Can you work these out from the model? Positions are in its coordinate system, mm. Round coordinates to 2 decimals unless told otherwise and drop trailing zeros. Loops run counter-clockwise (first coordinate to the right, second up) from the corner with the lowest first, then second, coordinate; pieces in that order, holes last. Notation, with made-up numbers: (46, -35.75) - (95, -35.75) arc R28 cw to (95, -12.75) - close; hole circle Ø11 at (-25.75, 59.25). An arc over 180 degrees is marked (long way). Answer as CSV lines item,"result".
```python
from build123d import *

# Parameters (mm, degrees)
F0_W     = 1219.2
F0_H     = 76.2
F1_DEPTH = 38.1
F3_DEPTH = 38.101
F4_R     = 5.08


with BuildPart() as f1:
    # F0 (on Top) → F1 (new body)
    with BuildSketch(Plane.XY):
        Rectangle(F0_W, F0_H)
    extrude(amount=F1_DEPTH)

    # F2 (on face) → F3 (cut, through all)
    with BuildSketch(Plane.XY.offset(38.1)):
        Polygon((-609.6, 38.1), (-609.6, -38.1), (-533.4, 38.1), align=None)
        Polygon((533.4, 38.1), (609.6, -38.1), (609.6, 38.1), align=None)
    extrude(amount=-F3_DEPTH, mode=Mode.SUBTRACT)

    # F4
    f4_edges = [f1.edges().sort_by_distance(p)[0] for p in [
        (0, 38.1, 0),
        (0, -38.1, 0),
        (0, -38.1, 38.1),
        (0, 38.1, 38.1),
    ]]
    fillet(f4_edges, radius=F4_R)


solid = f1.part
```
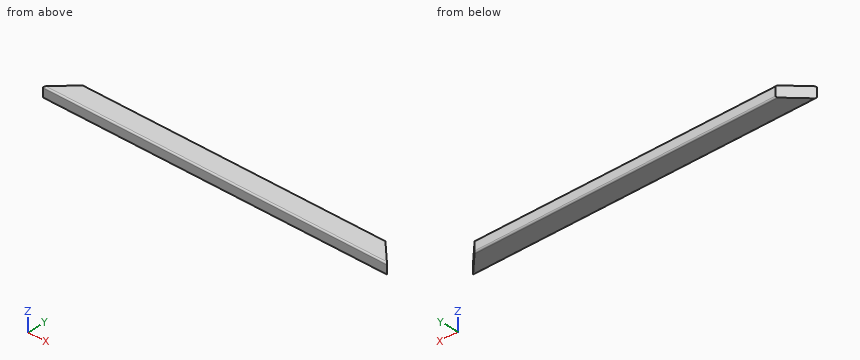
Q1. Imagine slicing it at B-B (y = -12). Write out the boundary of the cut face in (x, z).
Checks:
outline,"(-583.5, 0) - (583.5, 0) - (583.5, 38.1) - (-583.5, 38.1) - close"
Q2. I'm going to push flat-ended pins straight in: pin 1 Ø10 at (y, z) = (2.5, 14.5) entering from -X; pin 2 Ø2 at (y, z) = (13.5, 24.5) entering from -X; pin 3 Ø3 at (y, z) = (-19, 11) entering from -X. Where does each tip first touch, or does it pass through?
Checks:
pin 1,"x = -574"
pin 2,"x = -559"
pin 3,"x = -592"
Q3. If I drill on line 1 along Z through (x, y) = (58.5, -34.5); line 2 along X through (y, z) = (-11, 16.5); line 3 along X through (y, z) = (-4, 21), over which ranges is the centre line in solid material (lowest first)? Write a range as [from, to].
Checks:
line 1,"[0.22, 37.88]"
line 2,"[-582.5, 582.5]"
line 3,"[-575.5, 575.5]"
Q4. Imagine slicing it at A-A (z = 21.5). Write out the boundary of the cut face in (x, y), then the cut area to 3 significant figures.
Checks:
outline,"(-609.6, -38.1) - (609.6, -38.1) - (533.4, 38.1) - (-533.4, 38.1) - close"
area,"87,100 mm²"
